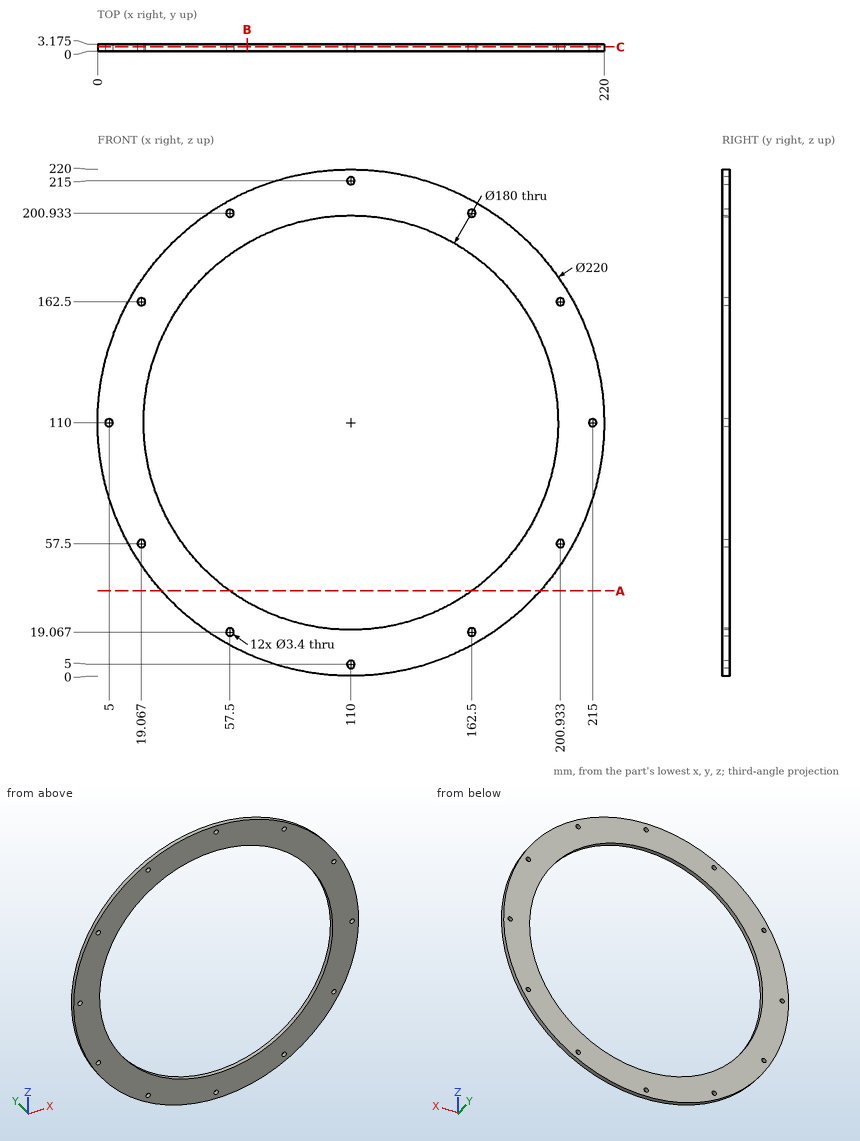
Print and shaded views of the part. All mm, measured from the part's lowest x, y and z. Give positions to 0.01 mm unless a question says otherwise; leave off trailing zeros. Write each loop counter-clockwise with the first axis right and the second up, starting at its lowest first coordinate (ties: lowest second). Pieces come first, ordered by that corner, then holes. Notation, with made-up numbers: (70.25, 7.25) - (129.25, 7.25) arc R21 ccw to (129.25, 19.25) - close; hole circle Ø2 at (-20.75, -19.75). An arc over 180 degrees is marked (long way). Put each result on its own line as item: value.
(1) Saw through at B-B (x = 65). List the corners of the cut face in (y, z) (1 decimal).
Working result:
outline: (0, 9.6) - (3.2, 9.6) - (3.2, 32.1) - (0, 32.1) - close; (0, 187.9) - (3.2, 187.9) - (3.2, 210.4) - (0, 210.4) - close
(2) Saw through at C-C (y = 1.95). Count the separate pieces of the cut face and the enclosed holes in it, then the cut area to 3 significant figures.
Working result:
separate pieces: 1
enclosed holes: 13
area: 12,500 mm^2
(3) Drop flat-ended pins along their axis: pin 1 Ø1.5 at (y, z) = (2, 150) entering from +X; pin 2 Ø1 at (y, z) = (1.5, 119) entering from +X. Give the stop position or say it passes through.
Working result:
pin 1: x = 212.76
pin 2: x = 219.67
(4) Wall check: L1, parallel to X at y = 1.75, z = 57.5; L2, parallel to X at y = 2, z = 19; L3, parallel to Z at x = 111, y = 1.95 (1 decimal). Give the ranges that are in metal, low to high.
Working result:
L1: 13.34 to 17.37, 20.77 to 36.9, 183.1 to 199.23, 202.63 to 206.66
L2: 48.2 to 55.8, 59.2 to 160.8, 164.2 to 171.8
L3: 0 to 3.6, 6.4 to 20, 200 to 213.6, 216.4 to 220
(5) Saw through at A-A (z = 37). List the corners of the cut face in (x, y) (1 decimal), then the cut area to 3 significant figures.
Working result:
outline: (27.7, 0) - (57.4, 0) - (57.4, 3.2) - (27.7, 3.2) - close; (162.6, 0) - (192.3, 0) - (192.3, 3.2) - (162.6, 3.2) - close
area: 188 mm^2
